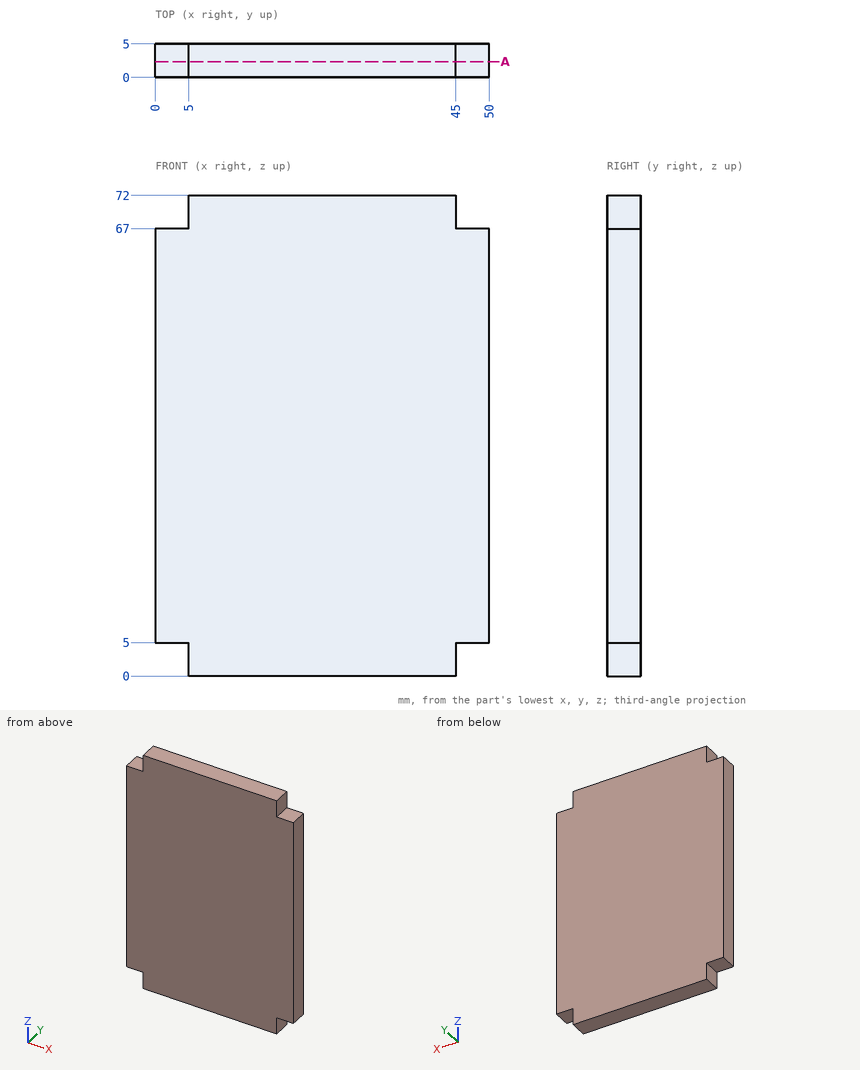
Source: three-view drawing plus pictorial views. Frame: mm from the lowest corner of the part. Give positions to 0.01 mm unless a question says otherwise; leave off trailing zeros. Loops run counter-clockwise (first coordinate to the right, second up) from the corner with the lowest first, then second, coordinate; pieces in that order, holes last.
1) Contact query for flat-ended pins moving along their axis: pin 1 (1.5 mm diameter, centred on y = 1.5, z = 3, fed in from +X); pin 2 (2.5 mm diameter, centred on x = 48, y = 3.5, fed in from -Z). Output: stop coordinate, or through.
A:
pin 1: stops at x = 45
pin 2: stops at z = 5
2) Section query A-A on y = 2.35. Return the cut outline in (x, z).
A:
outline: (0, 5) - (5, 5) - (5, 0) - (45, 0) - (45, 5) - (50, 5) - (50, 67) - (45, 67) - (45, 72) - (5, 72) - (5, 67) - (0, 67) - close
3) Line query: L1, parallel to X at y = 2.65, z = 69; L2, parallel to Z at x = 47, y = 4.3. Output: solid intervals per line, ascending.
A:
L1: x = 5 to 45
L2: z = 5 to 67
